from build123d import *

# Parameters (mm, degrees)
F0_R     = 1.825
F1_DEPTH = 1.5
F2_R     = 5


with BuildPart() as f1:
    # F0 (on Front) → F1 (new body)
    with BuildSketch(Plane.XZ):
        with BuildLine():
            Line((9.91, 0), (0, 0))
            Line((0, 0), (-9.91, 0))
            Line((-9.91, 0), (-9.91, -5.46))
            Line((-9.91, -5.46), (-7.858928, -8.658922))
            Line((-7.858928, -8.658922), (-7.858928, -15.258922))
            Line((-7.858928, -15.258922), (-9.91, -18.457845))
            Line((-9.91, -18.457845), (-9.91, -53.967845))
            Line((-9.91, -53.967845), (-6.083598, -59.467722))
            Line((-6.083598, -59.467722), (-2.257197, -53.967845))
            Line((-2.257197, -53.967845), (-2.257197, -22.297845))
            ThreePointArc((-2.257197, -22.297845), (0, -20.040648), (2.257197, -22.297845))
            Line((2.257197, -22.297845), (2.257197, -53.967845))
            Line((2.257197, -53.967845), (6.083598, -59.467722))
            Line((6.083598, -59.467722), (9.91, -53.967845))
            Line((9.91, -53.967845), (9.91, -18.457845))
            Line((9.91, -18.457845), (7.858928, -15.258922))
            Line((7.858928, -15.258922), (7.858928, -8.658922))
            Line((7.858928, -8.658922), (9.91, -5.46))
            Line((9.91, -5.46), (9.91, 0))
        make_face()
        with Locations((-6.705, -2.73)):
            Circle(F0_R, mode=Mode.SUBTRACT)
        with Locations((6.705, -2.73)):
            Circle(F0_R, mode=Mode.SUBTRACT)
    extrude(amount=-F1_DEPTH)

    # F2
    f2_edges = [f1.edges().sort_by_distance(p)[0] for p in [
        (7.858928, 0.75, -15.258922),
        (-7.858928, 0.75, -15.258922),
        (-7.858928, 0.75, -8.658922),
        (7.858928, 0.75, -8.658922),
        (9.91, 0.75, -53.967845),
        (2.257197, 0.75, -53.967845),
        (-9.91, 0.75, -53.967845),
        (-2.257197, 0.75, -53.967845),
    ]]
    fillet(f2_edges, radius=F2_R)


solid = f1.part
Geometry: final body of the model. Coordinates: model frame, mm. A direction names the side the tool comes from. Give positions to 0.01 mm unless a question says otherwise; leave off trailing zeros. Write each loop counter-clockwise with the first axis right and the second up, starting at its lowest first coordinate (ties: lowest second). Pieces come first, ordered by that corner, then holes. Notation, with made-up numbers: M -2.5,-36 L 56.5,-36 A8 cw 56.5,-28 Z; hole C -29.5,23.25 d10. An arc over 180 degrees is marked long. Answer in a Markdown table with one row per item. Add a question column.
(1) Reachability of faces 1 (the flat face through (-7.57, 0.74, -57.33)), 2 (the flat face through (4.598, 0.74, -57.332)), 3 (the cylindrical face through (-8.066, 0.76, -8.699)), 4 (the cylindrical face through (8.055, 0.76, -15.181)), 5 (the flat face through (0, 1, 0)) from +Z, -Z, +X, -X, +Y, -Y: full face, straight path, thin tool, end or side. Return the list, or none.
(2) Section D-D on x = 0. Return loops of the section in (y, z).
(3) Section B-B on y = 0.3. Return loops of the section in (x, z) (3 decimals), and give its area (3 significant figures).
(4) Mould query, pull axis Z, two halves, no side actions, for faces 6 (the flat face through (9.91, 1, -36)), 7 (the flat face through (-7.859, 1, -12)), 8 (the cylindrical face through (2.493, 0.76, -53.916)). Classes: +Z half, -Z half, draft (parallel to the pull), parting line (faces both ways), or undercut.
(5) Section A-A on z = -23. Return loops of the section in (x, y).
(6) Section C-C on z = -2.73. Return loops of the section in (x, y).
(7) Ray query, line 1 (X direction, y = 0.95, z = -46.5); line 2 (Z direction, x = 9.25, y = 0.85); line 3 (Z direction, x = -9, y = 0.7). Return the intervals inside material, ascending.
Result set:
| question | item | result |
|---|---|---|
| 1 | face 1 | -Z, -X, +Y, -Y |
| 1 | face 2 | -Z, +Y, -Y |
| 1 | face 3 | -X, +Y, -Y |
| 1 | face 4 | +X, +Y, -Y |
| 1 | face 5 | +Z, +X, -X, +Y, -Y |
| 2 | outline | M 0,-20.04 L 1.5,-20.04 L 1.5,0 L 0,0 Z |
| 3 | outline | M -9.91,-52.4 A5 ccw -9.014,-55.255 L -6.084,-59.468 L -3.153,-55.255 A5 ccw -2.257,-52.4 L -2.257,-22.298 A2.257 cw 2.257,-22.298 L 2.257,-52.4 A5 ccw 3.153,-55.255 L 6.084,-59.468 L 9.014,-55.255 A5 ccw 9.91,-52.4 L 9.91,-18.458 L 8.65,-16.492 A5 cw 7.859,-13.794 L 7.859,-10.124 A5 cw 8.65,-7.425 L 9.91,-5.46 L 9.91,0 L -9.91,0 L -9.91,-5.46 L -8.65,-7.425 A5 cw -7.859,-10.124 L -7.859,-13.794 A5 cw -8.65,-16.492 L -9.91,-18.458 Z; hole C -6.705,-2.73 d3.65; hole C 6.705,-2.73 d3.65 |
| 3 | area | 899 mm^2 |
| 4 | face 6 | draft |
| 4 | face 7 | undercut |
| 4 | face 8 | -Z half |
| 5 | outline | M -9.91,0 L -2.26,0 L -2.26,1.5 L -9.91,1.5 Z; M 2.26,0 L 9.91,0 L 9.91,1.5 L 2.26,1.5 Z |
| 6 | outline | M -9.91,0 L -8.53,0 L -8.53,1.5 L -9.91,1.5 Z; M -4.88,0 L 4.88,0 L 4.88,1.5 L -4.88,1.5 Z; M 8.53,0 L 9.91,0 L 9.91,1.5 L 8.53,1.5 Z |
| 7 | line 1 | x = -9.91 to -2.26, 2.26 to 9.91 |
| 7 | line 2 | z = -54.88 to -17.43, -6.49 to 0 |
| 7 | line 3 | z = -55.28 to -17.04, -6.88 to 0 |
